Input: part model. Units: mm. Frame: model coordinates. A direction names the side the tool comes from. Coordinates: 2 decimals unless noted, no trailing zeros. Loops run counter-clockwise (first coordinate to the right, second up) from the corner with the lowest first, then second, coordinate; pieces in that order, holes last.
```python
from build123d import *

# Parameters (mm, degrees)
F0_R     = 300
F1_DEPTH = 550
F2_R     = 200
F3_DEPTH = 150
F5_R     = 60
F6_DEPTH = 250
F4_R     = 100
F7_DEPTH = 400.001


with BuildPart() as f1:
    # F0 (on Top) → F1 (new body)
    with BuildSketch(Plane.XY):
        Circle(F0_R)
    extrude(amount=F1_DEPTH)

    # F2 (on face) → F3 (cut)
    with BuildSketch(Plane.XY.offset(550)):
        Circle(F2_R)
    extrude(amount=-F3_DEPTH, mode=Mode.SUBTRACT)

    # F5 (on face) → F6 (join)
    with BuildSketch(Plane(origin=(0, 0, 0), x_dir=(1, 0, 0), z_dir=(0, 0, -1))):
        with BuildLine():
            ThreePointArc((600, 80), (570.710678, 150.710678), (500, 180))
            Line((500, 180), (-500, 180))
            ThreePointArc((-500, 180), (-570.710678, 150.710678), (-600, 80))
            Line((-600, 80), (-600, -80))
            ThreePointArc((-600, -80), (-570.710678, -150.710678), (-500, -180))
            Line((-500, -180), (500, -180))
            ThreePointArc((500, -180), (570.710678, -150.710678), (600, -80))
            Line((600, -80), (600, 80))
        make_face()
        with Locations((-450, 0)):
            Circle(F5_R, mode=Mode.SUBTRACT)
        with Locations((450, 0)):
            Circle(F5_R, mode=Mode.SUBTRACT)
    extrude(amount=-F6_DEPTH)

    # F4 (on face) → F7 (cut, through all)
    with BuildSketch(Plane.XY.offset(400)):
        Circle(F4_R)
    extrude(amount=-F7_DEPTH, mode=Mode.SUBTRACT)


solid = f1.part
```
Item 1: Section query A-A (x = 450). Output: boundary loops of the cut face in (y, z), then the cut area to 3 significant figures.
Result:
outline: (-180, 0) - (-60, 0) - (-60, 250) - (-180, 250) - close; (60, 0) - (180, 0) - (180, 250) - (60, 250) - close
area: 60,000 mm2
Item 2: Section query C-C (y = 0). Output: boundary loops of the cut face in (x, z).
Result:
outline: (-600, 0) - (-510, 0) - (-510, 250) - (-600, 250) - close; (-390, 0) - (-100, 0) - (-100, 400) - (-200, 400) - (-200, 550) - (-300, 550) - (-300, 250) - (-390, 250) - close; (100, 0) - (390, 0) - (390, 250) - (300, 250) - (300, 550) - (200, 550) - (200, 400) - (100, 400) - close; (510, 0) - (600, 0) - (600, 250) - (510, 250) - close
Item 3: Contact query for flat-ended pins moving along their axis: P1, Ø8, axis at x = -74.5, z = 164, coming from the -Y side; P2, Ø6, axis at x = 263, z = 309, coming from the +Y side; P3, Ø8, axis at y = 173, z = 457.5, coming from the -X side. Output: stop coordinate, or through.
Result:
P1: stops at y = -291.6
P2: stops at y = 149.67
P3: stops at x = -247.87
Item 4: Line query: L1, parallel to Y at x = -450, z = 59; L2, parallel to Y at x = 0, z = 163.5; L3, parallel to Z at x = 299, y = -162.5. Output: solid intervals per line, ascending.
Result:
L1: y = -180 to -60, 60 to 180
L2: y = -300 to -100, 100 to 300
L3: z = 0 to 250
Item 5: Section query B-B (z = 108.5). Output: boundary loops of the cut face in (x, y), then the cut area to 3 significant figures.
Result:
outline: (-600, -80) arc R100 ccw to (-500, -180) - (-240, -180) arc R300 ccw to (240, -180) - (500, -180) arc R100 ccw to (600, -80) - (600, 80) arc R100 ccw to (500, 180) - (240, 180) arc R300 ccw to (-240, 180) - (-500, 180) arc R100 ccw to (-600, 80) - close; hole circle Ø120 at (-450, 0); hole circle Ø200 at (0, 0); hole circle Ø120 at (450, 0)
area: 450,000 mm2
Item 6: Mould query, pull axis Y, two halves, no side actions, for faces 1 (the face through (-569.929, -151.484, 123.25)), 2 (the face through (-8, 129, 0)), 3 (the face through (190.764, 60.075, 476.05)). Classes: +Y half, -Y half, draft (parallel to the pull), parting line (faces both ways), or undercut.
Result:
face 1: -Y half
face 2: draft
face 3: undercut
Item 7: Reachability of faces 4 (the face through (368, 180, 123)), 5 (the face through (-368, -180, 123)), 6 (the face through (-299.71, 13.19, 271.15)) from +Z, -Z, +X, -X, +Y, -Y: full face, straight path, thin tool, end or side. Return the list, or none.
Result:
face 4: +Z, -Z, +X, +Y
face 5: +Z, -Z, -X, -Y
face 6: +Z
Item 8: Section query D-D (y = -124.5). Output: boundary loops of the cut face in (x, z), then the cut area to 3 significant figures.
Result:
outline: (-589.55, 0) - (589.55, 0) - (589.55, 250) - (272.95, 250) - (272.95, 550) - (156.52, 550) - (156.52, 400) - (-156.52, 400) - (-156.52, 550) - (-272.95, 550) - (-272.95, 250) - (-589.55, 250) - close
area: 412,000 mm2
